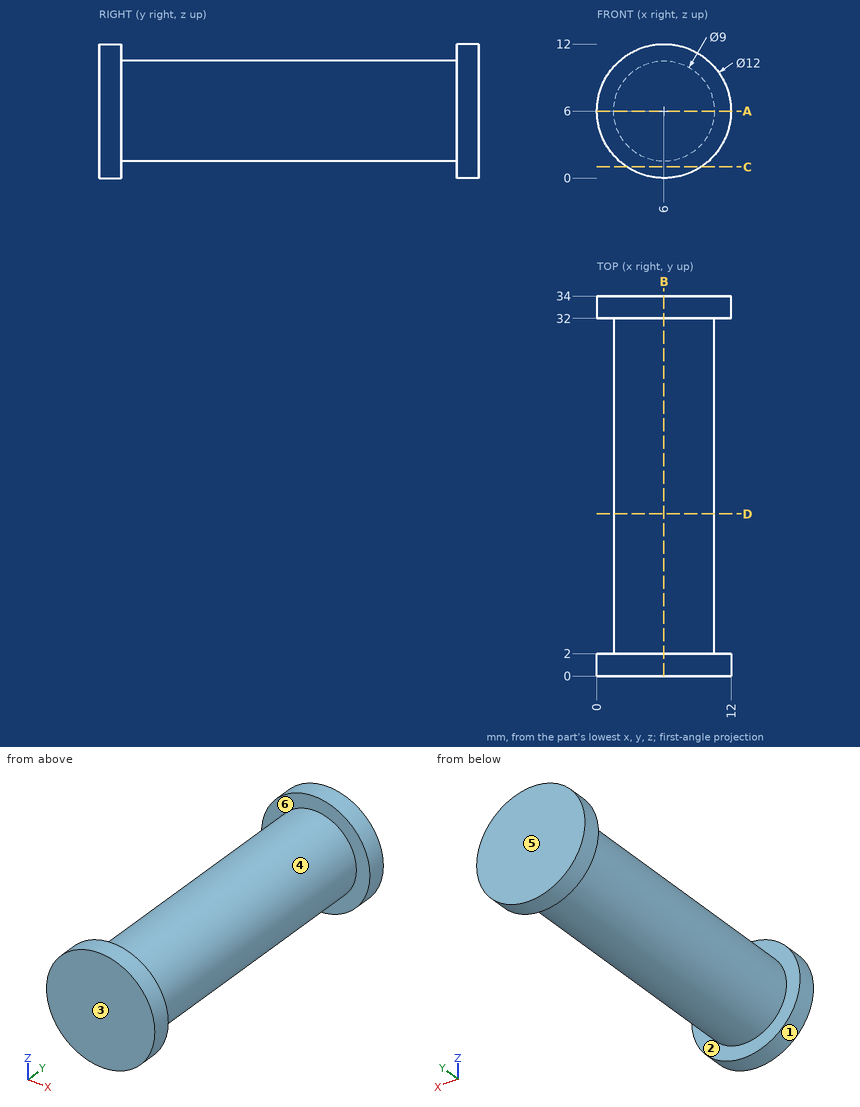
Study the drawing (mm; zero at the part's minimum x, y, z) and answer. A direction names the side the tool comes from. Round coordinates to 2 decimals unless told otherwise and drop trailing zeros. Write each loop counter-clockwise with the first axis right and the second up, starting at its lowest first coordinate (ties: lowest second). Pieces come first, ordered by that corner, then holes. Notation, with made-up numbers: (75.25, -27) - (95.25, -27) arc R10 cw to (95.25, -15) - close; hole circle Ø9 at (-34.5, 56.25). An arc over 180 degrees is marked (long way). Use a Markdown table: item, result. Add a question column.
1. The part is cut by section D-D (y = 14.5). Write down the section's boundary in (x, z).
2. Consider line 1 (Y direction, x = 6.5, z = 11); line 2 (Z direction, x = 5.75, y = 18); line 3 (Z direction, x = 3.25, y = 8). Determine where each line is inside the solid, lowest interval first.
3. The part is cut by section A-A (z = 6). Write down the section's boundary in (x, y).
4. A tool of negligible diameter and unlimited length cuts with its end or side. For the marked faces 5 and 6, from which of +Z, -Z, +X, -X, +Y, -Y can it reach the whole face along a straight path? Write none if from no direction.
5. Flat-ended cylindrical pins translate along their axes: P1, Ø1, axis at y = 27.5, z = 7.5, coming from the +X side; P2, Ø3, axis at x = 8.5, y = 27, coming from the -Z side; P3, Ø3, axis at x = 2.5, y = 6.5, coming from the +Z side. Find the tip coordinate at first contact, or state that the pin passes through.
6. The part is cut by section B-B (x = 6). Write down the section's boundary in (y, z).
7. The part is cut by section C-C (z = 1). Write down the section's boundary in (x, y).
8. For a pull along Y with two mould halves and no side action, classify the marked faces 1, 2, 3 and 4 as +Y half, -Y half, draft (parallel to the pull), parting line (faces both ways), or undercut.
Reported:
| question | item | result |
|---|---|---|
| 1 | outline | circle Ø9 at (6, 6) |
| 2 | line 1 | 0 to 2, 32 to 34 |
| 2 | line 2 | 1.51 to 10.49 |
| 2 | line 3 | 2.44 to 9.56 |
| 3 | outline | (0, 0) - (12, 0) - (12, 2) - (10.5, 2) - (10.5, 32) - (12, 32) - (12, 34) - (0, 34) - (0, 32) - (1.5, 32) - (1.5, 2) - (0, 2) - close |
| 4 | face 5 | +Z, -Z, +X, -X, +Y |
| 4 | face 6 | none |
| 5 | P1 | x = 10.39 |
| 5 | P2 | z = 1.61 |
| 5 | P3 | z = 10.03 |
| 6 | outline | (0, 0) - (2, 0) - (2, 1.5) - (32, 1.5) - (32, 0) - (34, 0) - (34, 12) - (32, 12) - (32, 10.5) - (2, 10.5) - (2, 12) - (0, 12) - close |
| 7 | outline | (2.68, 0) - (9.32, 0) - (9.32, 2) - (2.68, 2) - close; (2.68, 32) - (9.32, 32) - (9.32, 34) - (2.68, 34) - close |
| 8 | face 1 | draft |
| 8 | face 2 | undercut |
| 8 | face 3 | -Y half |
| 8 | face 4 | undercut |
